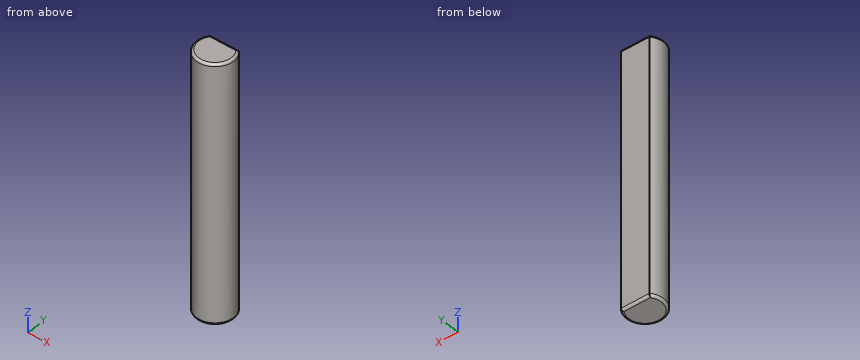
Autodesk Inventor part; units mm, degrees
ref_plane "YZ Plane" through (0, 0, 0) normal (1, 0, 0) x (0, 1, 0)
ref_plane "XZ Plane" through (0, 0, 0) normal (0, 1, 0) x (-1, 0, 0)
ref_plane "XY Plane" through (0, 0, 0) normal (0, 0, 1) x (1, 0, 0)
sketch "Sketch1" plane through (0, 0, 0) normal (0, 0, 1) x (1, 0, 0)
  circle A0 centre (0, 0) radius 4
  line L0 (-3.1225, 2.5) -> (3.1225, 2.5)
  dimension "d0" = 8
  dimension "d1" = 2.5
extrude "Extrusion1" add sketch "Sketch1" along normal blind 55 contours A0 L0 picked at (-0.7341, 0.0257)
fillet "Fillet1" radius 0.5 4 edges at (0, -4, 55) (0, 2.5, 55) (0, -4, 0) (0, 2.5, 0)
properties part number "8mm D-Shaft axle (3d print)"
Geometry check sheet. Reference: the model listing, model coordinates, mm. Give positions to 0.01 mm unless a question says otherwise; leave off trailing zeros. Write each loop counter-clockwise with the first axis right and the second up, starting at its lowest first coordinate (ties: lowest second). Pieces come first, ordered by that corner, then holes.
1) Go/stop test with a flat-tipped pin: pin 1 Ø1 at (x, z) = (-0.5, 13.5) entering from -Y. Record where the tip stops, or that it passes through.
Values follow:
pin 1: stops at y = -4
2) Thickness scan on line 1 (X direction, y = -0.25, z = 26); line 2 (X direction, y = 2.25, z = 22); line 3 (Y direction, x = 2.5, z = 14). Record the ranges inside material, lowest first.
Values follow:
line 1: x = -3.99 to 3.99
line 2: x = -3.31 to 3.31
line 3: y = -3.12 to 2.5
3) Cross-section at A-A (z = 13). Record the boundary of the cut face in (x, y).
Values follow:
outline: (-3.12, 2.5) arc R4 ccw (long way) to (3.12, 2.5) - close
